Verification items for the finished model (mm, model axes). A direction names the side the tool comes from. Give positions to 0.01 mm unless a question says otherwise; leave off trailing zeros. Write each loop counter-clockwise with the first axis right and the second up, starting at its lowest first coordinate (ties: lowest second). Pieces come first, ordered by that corner, then holes.
Autodesk Inventor part; units mm, degrees
ref_plane "YZ Plane" through (0, 0, 0) normal (1, 0, 0) x (0, 1, 0)
ref_plane "XZ Plane" through (0, 0, 0) normal (0, 1, 0) x (-1, 0, 0)
ref_plane "XY Plane" through (0, 0, 0) normal (0, 0, 1) x (1, 0, 0)
sketch "Sketch1" plane through (0, 0, 0) normal (0, 0, 1) x (1, 0, 0)
  line L0 (0, 0) -> (0, 5.657)
  line L1 (2.8285, 3.4285) -> (2.2285, 3.4285)
  line L2 (2.8285, 2.2285) -> (2.2285, 2.2285)
  line L3 (2.2285, 3.4285) -> (2.8285, 3.4285)
  line L4 (2.8285, 2.2285) -> (2.2285, 2.2285)
  line L5 (2.2285, 3.4285) -> (4, 3.4285)
  line L6 (4, 2.2285) -> (2.8285, 2.2285)
  line L7 (2.2285, 3.4285) -> (4, 3.4285)
  line L8 (2.2285, 3.4285) -> (4, 3.4285)
  line L9 (0, -2.1715) -> (0, 0)
  line L10 (0, 5.657) -> (0, 6.8285)
  line L11 (8, -2.1715) -> (8, 6.8285)
  line L12 (4, 3.4285) -> (4, 3.4285)
  line L13 (4, 3.4285) -> (4, 2.2285)
  line L14 (4, 2.2285) -> (4, 2.2285)
  line L15 (8, -2.1715) -> (8, -4.1715)
  line L16 (8, -4.1715) -> (0, -4.1715)
  line L17 (2.2285, 3.4285) -> (1.9283, 3.4285)
  line L18 (1.9283, 3.4285) -> (0, 5.3568)
  line L19 (2.2285, 2.2285) -> (1.9283, 2.2285)
  line L20 (1.9283, 2.2285) -> (0, 0.3002)
  line L21 (0, -2.1715) -> (0, -4.1715)
  line L22 (4, 2.8285) -> (8, 2.8285) construction
  line L23 (8, 6.8285) -> (8, 11.8285)
  line L24 (8, 11.8285) -> (0, 11.8285)
  line L25 (0, 11.8285) -> (0, 6.8285)
  line L26 (8, 11.8285) -> (10, 11.8285)
  line L27 (10, 11.8285) -> (10, -4.1715)
  line L28 (10, -4.1715) -> (8, -4.1715)
  line L29 (10, 11.8285) -> (7, 11.8285) construction
  line L30 (10, 11.8285) -> (5, 11.8285) construction
  line L31 (5, 11.8285) -> (5, 6.7848) construction
  point P0 (4.938, 0.6604)
  point P1 (0.4, 0.4)
  point P2 (0.4, 5.257)
  point P3 (0.4, -2.1715)
  point P4 (0.25, 5.407)
  point P5 (0.25, -2.1715)
  point P6 (0.25, -4.1715)
  dimension "d11" = 8
  dimension "d23" = 4
  dimension "d24" = 7
  dimension "d25" = 5
  dimension "d26" = 2
  dimension "d29" = 5
  dimension "d78" = 4
extrude "Extrusion1" add sketch "Sketch1" against normal blind 71 contours L0 L20 L19 L2 L6 L13 L5 L1 L17 L18 L10 L25 L24 L23 L11 L15 L16 L21 L9 | L15 L11 L23 L26 L27 L28
sketch "Sketch2" plane through (0, 0, 0) normal (0, 0, 1) x (1, 0, 0)
  line L0 (10, -4.1715) -> (10, 11.8285) construction
  line L1 (10, 11.8285) -> (5, 11.8285) construction
  line L2 (10, 11.8285) -> (0, 11.8285) construction
  line L3 (5, 11.8285) -> (5, 6.8285) construction
  point P0 (0, 0)
  dimension "d30" = 5
hole "Hole1" at (5, 6.8285, 0) direction (0, 0, -1) diameter 1.567 depth 8 tip angle 118
sketch "Sketch3" plane through (0, 0, -71) normal (0, 0, -1) x (-1, 0, 0)
  line L0 (-10, 11.8285) -> (-10, -4.1715) construction
  line L1 (-10, 11.8285) -> (-5, 11.8285) construction
  line L2 (0, 11.8285) -> (-10, 11.8285) construction
  line L3 (-5, 11.8285) -> (-5, 6.8285) construction
  circle A0 centre (-5, 6.8285) radius 0.7835 construction
  point P0 (0, 0)
  dimension "d38" = 5
  dimension "d40" = 5
hole "Hole2" at (5, 6.8285, -71) direction (0, 0, 1) diameter 1.567 depth 8 tip angle 118
chamfer "Chamfer1" distance 0.3 angle 45 1 edges at (5, 7.612, 0)
chamfer "Chamfer2" distance 0.3 angle 45 1 edges at (5, 6.045, -71)
sketch "Sketch4" plane through (0, -4.1715, 0) normal (0, -1, 0) x (1, 0, 0)
  line L0 (0, 0) -> (0, -71) construction
  line L1 (0, 0) -> (0, -10) construction
  line L2 (0, -10) -> (0, -35.5) construction
  line L3 (0, -71) -> (0, -61) construction
  line L4 (0, -35.5) -> (10, -35.5) construction
  line L5 (10, 0) -> (10, -71) construction
  line L6 (0, -61) -> (10, -61) construction
  line L7 (0, -10) -> (10, -10) construction
  line L8 (0, -71) -> (6, -71)
  line L9 (6, -71) -> (6, 0)
  point P0 (5, 0)
  point P1 (5, -71)
  point P2 (6, -61)
  point P3 (6, -35.5)
  point P4 (6, -10)
  dimension "d54" = 10
  dimension "d55" = 10
  dimension "d63" = 6
  dimension "d64" = 35.5
hole "Hole3" at (6, -4.1715, -10) at (6, -4.1715, -35.5) at (6, -4.1715, -61) direction (0, 1, 0) diameter 1.567 end through all
sketch "Sketch5" plane through (0, 11.8285, 0) normal (0, 1, 0) x (1, 0, 0)
  point P0 (0, 0)
chamfer "Chamfer3" distance 0.3 angle 45 1 edges at (6, -4.1715, -9.2165)
chamfer "Chamfer4" distance 0.3 angle 45 2 edges at (6, -4.1715, -34.7165) (6, -4.1715, -60.2165)
sketch "Sketch6" plane through (0, 11.8285, 0) normal (0, 1, 0) x (1, 0, 0)
  line L0 (0, 0) -> (10, 0)
  line L1 (4, 71) -> (4.3098, 49.0022) construction
  line L2 (5, 0) -> (4.6902, 21.9978) construction
  point P0 (5, 61.7835)
  dimension "d71" = 22
  dimension "d72" = 22
sketch "Sketch7" plane through (0, 11.8285, 0) normal (0, 1, 0) x (1, 0, 0)
  line L0 (0, 0) -> (10, 0)
  line L1 (0, 0) -> (7.5, 0)
  line L2 (7.5, 0) -> (7.5, 20)
  line L3 (0, 71) -> (10, 71)
  line L4 (0, 71) -> (7.5, 71)
  line L5 (7.5, 71) -> (7.5, 51)
  dimension "d73" = 7.5
  dimension "d74" = 20
  dimension "d76" = 7.5
  dimension "d77" = 20
sketch "Sketch8" plane through (0, 11.8285, 0) normal (0, 1, 0) x (1, 0, 0)
  line L0 (0, 0) -> (6, 0)
  line L1 (10, 0) -> (0, 0)
  line L2 (6, 0) -> (6, 22)
  line L3 (0, 71) -> (6, 71)
  line L4 (10, 71) -> (0, 71)
  line L5 (6, 71) -> (6, 49)
  dimension "d79" = 6
  dimension "d80" = 22
  dimension "d81" = 6
  dimension "d82" = 22
hole "Hole4" at (6, 11.8285, -49) at (6, 11.8285, -22) direction (0, -1, 0) diameter 2 end through all
chamfer "Chamfer5" distance 0.3 angle 45 2 edges at (6, 11.8285, -50) (6, 11.8285, -23)
properties part number "Guide" material "Steel, Carbon"
Item 1: Scan lines: line 1 along Z through (x, y) = (6, 2.5); line 2 along X through (y, z) = (0, -10); line 3 along Y through (x, z) = (3.5, -19.5). Record each from-to range of solid material in increasing order.
Answer key:
line 1: z = -71 to -61.78, -60.22 to -50, -48 to -36.28, -34.72 to -23, -21 to -10.78, -9.22 to 0
line 2: x = 0 to 5.22, 6.78 to 10
line 3: y = -4.17 to 2.23, 3.43 to 11.83
Item 2: Sectioned sample at B-B on z = -10. Record the cut outline in (x, y), then the cut area to 3 significant figures.
Answer key:
outline: (0, -4.17) - (4.92, -4.17) - (5.22, -3.87) - (5.22, 11.83) - (0, 11.83) - (0, 5.36) - (1.93, 3.43) - (4, 3.43) - (4, 2.23) - (1.93, 2.23) - (0, 0.3) - close; (6.78, -3.87) - (7.08, -4.17) - (10, -4.17) - (10, 11.83) - (6.78, 11.83) - close
area: 126 mm2
Item 3: Depth check by flat-ended pin: pin 1 (1.3 mm diameter, centred on x = 6, z = -61, fed in from +Y); pin 2 (1.4 mm diameter, centred on x = 5, y = 6.83, fed in from -Z); pin 3 (1 mm diameter, centred on y = 3, z = -23.5, fed in from -X); pin 4 (0.9 mm diameter, centred on x = 5, y = 6.83, fed in from -Z). Enter the tip coordinate at first touch or a pass-through.
Answer key:
pin 1: passes through
pin 2: stops at z = -62.95
pin 3: stops at x = 1.86
pin 4: stops at z = -62.8
Item 4: Sectioned sample at D-D on z = -49. Record the cut outline in (x, y).
Answer key:
outline: (0, -4.17) - (5, -4.17) - (5, 11.53) - (4.7, 11.83) - (0, 11.83) - (0, 5.36) - (1.93, 3.43) - (4, 3.43) - (4, 2.23) - (1.93, 2.23) - (0, 0.3) - close; (7, -4.17) - (10, -4.17) - (10, 11.83) - (7.3, 11.83) - (7, 11.53) - close
Item 5: Release check for a two-part mould opening along Y. For faces 3 (the face through (5, 11.828, -35)), 4 (the face through (4.765, 7.576, -66.796)), 5 (the face through (5, 4, -71)) record: released by +Y, released by -Y, zero draft, split by the parting line, or undercut.
Answer key:
face 3: released by +Y
face 4: undercut
face 5: zero draft
Item 6: Sectioned sample at A-A on y = -1.75. Record the cut outline in (x, z).
Answer key:
outline: (0, -71) - (10, -71) - (10, 0) - (0, 0) - close; hole circle Ø2 at (6, -49); hole circle Ø2 at (6, -22); hole circle Ø1.57 at (6, -61); hole circle Ø1.57 at (6, -35.5); hole circle Ø1.57 at (6, -10)
Item 7: Sectioned sample at C-C on z = -24.5. Record the cut outline in (x, y), then the cut area to 3 significant figures.
Answer key:
outline: (0, -4.17) - (10, -4.17) - (10, 11.83) - (0, 11.83) - (0, 5.36) - (1.93, 3.43) - (4, 3.43) - (4, 2.23) - (1.93, 2.23) - (0, 0.3) - close
area: 151 mm2
Item 8: Set-up check for faces 1 (the face through (0, -2, -35)), 2 (the face through (1, 1.3, -35)): record each of +Z, -Z, +X, -X, +Y, -Y from which the full face is reachable in a straight line by a thin tool's end or side.
Answer key:
face 1: +Z, -Z, -X, +Y, -Y
face 2: +Z, -Z, -X
